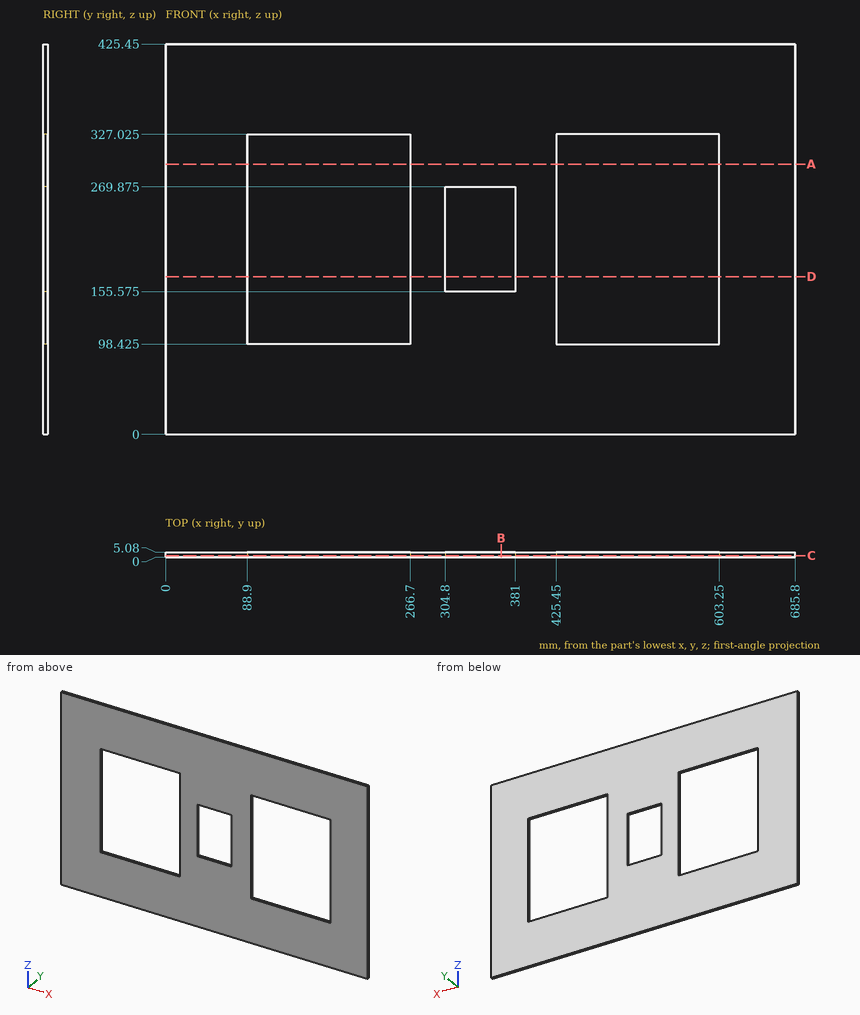
Print and shaded views of the part. All mm, measured from the part's lowest x, y and z. Give positions to 0.01 mm unless a question says otherwise; leave off trailing zeros. Write each loop counter-clockwise with the first axis right and the second up, starting at its lowest first coordinate (ties: lowest second). Pieces come first, ordered by that corner, then holes. Notation, with made-up numbers: (84.5, 29) -> (104.5, 29) arc R31 ccw to (104.5, 55) -> close; hole circle Ø10 at (60, 59). An arc over 180 degrees is marked (long way). Write item = value, one per line.
(1) Slice it at A-A, the plane z = 294.5. Give the cut face in (x, y), then the cut area to 3 significant figures.
Determined:
outline = (0, 0) -> (88.9, 0) -> (88.9, 5.08) -> (0, 5.08) -> close; (266.7, 0) -> (425.45, 0) -> (425.45, 5.08) -> (266.7, 5.08) -> close; (603.25, 0) -> (685.8, 0) -> (685.8, 5.08) -> (603.25, 5.08) -> close
area = 1,680 mm2
(2) Slice it at C-C, the plane y = 1.6. Give the cut face in (x, z) (3 decimals).
Determined:
outline = (0, 0) -> (685.8, 0) -> (685.8, 425.45) -> (0, 425.45) -> close; hole (88.9, 98.425) -> (266.7, 98.425) -> (266.7, 327.025) -> (88.9, 327.025) -> close; hole (304.8, 155.575) -> (381, 155.575) -> (381, 269.875) -> (304.8, 269.875) -> close; hole (425.45, 98.425) -> (603.25, 98.425) -> (603.25, 327.025) -> (425.45, 327.025) -> close
(3) Probe line 1 along X through (y, z) = (3.6, 177.5); line 2 along X through (y, z) = (0.9, 133.5); line 3 along Z through (x, y) = (595, 4.3) (3 decimals). List the from-to ranges inside material, lowest first.
Determined:
line_1 = 0 to 88.9, 266.7 to 304.8, 381 to 425.45, 603.25 to 685.8
line_2 = 0 to 88.9, 266.7 to 425.45, 603.25 to 685.8
line_3 = 0 to 98.425, 327.025 to 425.45
(4) Slice it at B-B, the plane x = 365.5. Give the cut face in (y, z) (3 decimals), then the cut area to 3 significant figures.
Determined:
outline = (0, 0) -> (5.08, 0) -> (5.08, 155.575) -> (0, 155.575) -> close; (0, 269.875) -> (5.08, 269.875) -> (5.08, 425.45) -> (0, 425.45) -> close
area = 1,580 mm2
(5) Slice it at D-D, the plane z = 172. Give the cut face in (x, y), then the cut area to 3 significant figures.
Determined:
outline = (0, 0) -> (88.9, 0) -> (88.9, 5.08) -> (0, 5.08) -> close; (266.7, 0) -> (304.8, 0) -> (304.8, 5.08) -> (266.7, 5.08) -> close; (381, 0) -> (425.45, 0) -> (425.45, 5.08) -> (381, 5.08) -> close; (603.25, 0) -> (685.8, 0) -> (685.8, 5.08) -> (603.25, 5.08) -> close
area = 1,290 mm2
